```python
from build123d import *

# Parameters (mm, degrees)
SKETCH1_R               = 20
BOSS_EXTRUDE1_DEPTH     = 25
SKETCH4_R               = 20
SKETCH4_R_2             = 17
CUT_EXTRUDE1_DEPTH      = 8
CUT_EXTRUDE2_REACH      = 39.749
CUT_EXTRUDE2_END_RADIUS = 17
SKETCH5_R               = 1.5


with BuildPart() as part:
    # Sketch1 → Boss-Extrude1 (new, symmetric)
    with BuildSketch(Plane.XY):
        Circle(SKETCH1_R)
    extrude(amount=BOSS_EXTRUDE1_DEPTH, both=True)

    # Sketch3 → Hole1 (revolve, cut)
    with BuildSketch(Plane(origin=(0, 0, 25), x_dir=(0, -1, 0), z_dir=(1, 0, 0))):
        Polygon((0, 0), (0, 56.609466809), (11, 50), (11, 9), (14, 9), (14, 0), align=None)
    hole1 = revolve(axis=Axis((0, 0, 36.310875039), (0, 0, -1)), mode=Mode.SUBTRACT)

    # Sketch4 → Cut-Extrude1 (cut)
    with BuildSketch(Plane.XY.offset(25)):
        Circle(SKETCH4_R)
        Circle(SKETCH4_R_2, mode=Mode.SUBTRACT)
    cut_extrude1 = extrude(amount=-CUT_EXTRUDE1_DEPTH, mode=Mode.SUBTRACT)

    # Mirror2: Hole1, Cut-Extrude1 across plane
    add(hole1.mirror(Plane.XY), mode=Mode.SUBTRACT)
    add(cut_extrude1.mirror(Plane.XY), mode=Mode.SUBTRACT)

    # Cut-Extrude2: up to this cylinder (the profile starts inside it)
    cut_extrude2_end = Plane(origin=(0, 0, 0), z_dir=(0, 0, 1)) * Cylinder(CUT_EXTRUDE2_END_RADIUS, 156.498, mode=Mode.PRIVATE)
    # Sketch5 → Cut-Extrude2 (cut, up to the surface)
    with BuildSketch(Plane(origin=(0, 0, 0), x_dir=(0, 0, -1), z_dir=(1, 0, 0)), mode=Mode.PRIVATE) as cut_extrude2_sk1:
        with Locations(Location((-21, 0, 0), (0, 0, 180))):
            Circle(SKETCH5_R)
    cut_extrude2_tool1 = extrude(cut_extrude2_sk1.sketch, amount=CUT_EXTRUDE2_REACH, mode=Mode.PRIVATE) & cut_extrude2_end
    add(cut_extrude2_tool1.solids().sort_by_distance((0, 0, 21))[0], mode=Mode.SUBTRACT)
    # Sketch5 → Cut-Extrude2 (cut, up to the surface)
    with BuildSketch(Plane(origin=(0, 0, 0), x_dir=(0, 0, -1), z_dir=(1, 0, 0)), mode=Mode.PRIVATE) as cut_extrude2_sk2:
        with Locations(Location((21, 0, 0), (0, 0, 180))):
            Circle(SKETCH5_R)
    cut_extrude2_tool2 = extrude(cut_extrude2_sk2.sketch, amount=CUT_EXTRUDE2_REACH, mode=Mode.PRIVATE) & cut_extrude2_end
    add(cut_extrude2_tool2.solids().sort_by_distance((0, 0, -21))[0], mode=Mode.SUBTRACT)


solid = part.part
```
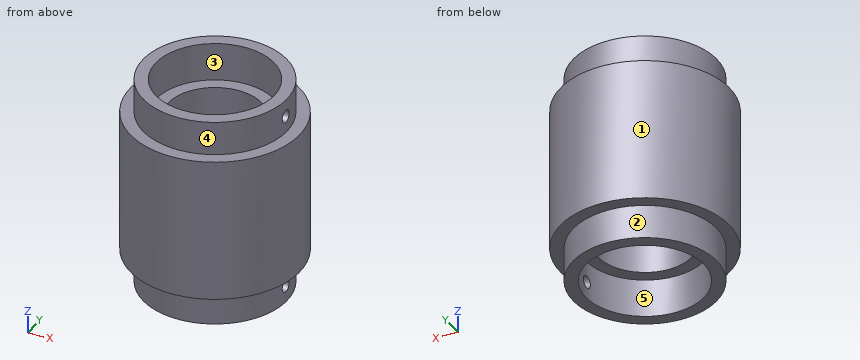
The model under review builds one solid part; all positions refer to its coordinate system, in mm. Face numbers are marked on the shaded views. A direction names the side the tool comes from. Round coordinates to 2 decimals unless told otherwise and drop trailing zeros. Write each loop counter-clockwise with the first axis right and the second up, starting at its lowest first coordinate (ties: lowest second). Pieces come first, ordered by that corner, then holes. Notation, with made-up numbers: (85.5, 1.5) - (123.5, 1.5) arc R20 cw to (123.5, 13.5) - close; hole circle Ø2 at (-33, 87). An arc over 180 degrees is marked (long way). Answer as CSV lines item,"result". Start each with the question number.
(1) Draft analysis for pull direction X (two halves, no side actions). For the marked faces 4 and 5, state which applies: pulls with the +X half, pulls with the -X half, needs draft (parallel to the pull), parting line crosses it, or undercut.
(2) We need section C-C on y = -5.5. State the section outline as (x, z) points.
(3) We need section B-B on x = 0. State the section outline as (y, z) points, plus the area to 3 significant figures.
(4) To check wall thickness, follow line 1 (Z direction, x = 15.95, y = 0); line 2 (Y direction, x = 0, z = 2.5); line 3 (Z direction, x = -10, y = 16). State the ranges of each line that lie inside material, in increasing order.
(5) For the marked faces 1, 2 and 3, list the 3-axis set-ups (+Z, -Z, +X, -X, +Y, -Y) from which the entire face can be reached by the end or side of a thin tool; tool diameter is ignored.
(6) For pin 1 Ø8 at (x, z) = (-8, -8) entering from +Y; pin 2 Ø10 at (y, z) = (11, -17.5) entering from -X; pin 3 Ø8 at (y, z) = (-8.5, 18) entering from -X, all flat-tipped, find the tip position at first contact; note any pin that passes through.
(7) We need section A-A on y = 0. Give the number of separate pieces and of enclosed holes in the cut face, plus the area to 3 significant figures.
(8) We need section D-D on z = 7.5. State the section outline as (x, y) points, plus the area to 3 significant figures.
Worked answers:
1,face 4,"parting line crosses it"
1,face 5,"undercut"
2,outline,"(-19.23, -17) - (-16.09, -17) - (-16.09, -25) - (-12.87, -25) - (-12.87, -16) - (-9.53, -16) - (-9.53, 16) - (-12.87, 16) - (-12.87, 25) - (-16.09, 25) - (-16.09, 17) - (-19.23, 17) - close; (9.53, -16) - (12.87, -16) - (12.87, -25) - (16.09, -25) - (16.09, -17) - (19.23, -17) - (19.23, 17) - (16.09, 17) - (16.09, 25) - (12.87, 25) - (12.87, 16) - (9.53, 16) - close"
3,outline,"(-20, -17) - (-17, -17) - (-17, -25) - (-14, -25) - (-14, -16) - (-11, -16) - (-11, 16) - (-14, 16) - (-14, 25) - (-17, 25) - (-17, 17) - (-20, 17) - close; (11, -16) - (14, -16) - (14, -25) - (17, -25) - (17, -17) - (20, -17) - (20, 17) - (17, 17) - (17, 25) - (14, 25) - (14, 16) - (11, 16) - close"
3,area,"696 mm²"
4,line 1,"-25 to -22.5, -19.5 to 19.5, 22.5 to 25"
4,line 2,"-20 to -11, 11 to 20"
4,line 3,"-17 to 17"
5,face 1,"+Z, -Z"
5,face 2,"-Z"
5,face 3,"+Z"
6,pin 1,"y = 19.6"
6,pin 2,"x = -19.07"
6,pin 3,"x = -19.46"
7,separate pieces,"4"
7,enclosed holes,"0"
7,area,"678 mm²"
8,outline,"circle Ø40 at (0, 0); hole circle Ø22 at (0, 0)"
8,area,"877 mm²"
